Here's how the part is built. I have some questions about the finished solid (model axes, mm). Face numbers are marked on the shaded views. A direction names the side the tool comes from. Coordinates: 2 decimals unless noted, no trailing zeros. Write each loop counter-clockwise with the first axis right and the second up, starting at its lowest first coordinate (ties: lowest second). Pieces come first, ordered by that corner, then holes.
from build123d import *

# Parameters (mm, degrees)
SKETCH1_W             = 44
SKETCH1_H             = 44
BOSS_EXTRUDE1_DEPTH   = 1.2
SKETCH2_W             = 23
SKETCH2_H             = 16
BOSS_EXTRUDE2_DEPTH   = 25
SKETCH3_W             = 7.6
SKETCH3_H             = 10
BOSS_EXTRUDE3_DEPTH   = 10
FILLET1_R             = 1
SKETCH4_W             = 15
SKETCH4_H             = 7.6
BOSS_EXTRUDE4_DEPTH   = 10
CHAMFER2_SIZE         = 3
CHAMFER2_SIZE2        = 0.528980942
CHAMFER2_PART_2_SIZE  = 3
CHAMFER2_PART_2_SIZE2 = 0.528980942
CHAMFER2_PART_3_SIZE  = 3
CHAMFER2_PART_3_SIZE2 = 0.528980942
CHAMFER1_SIZE         = 4
CHAMFER1_SIZE2        = 1.455880937
CHAMFER1_PART_2_SIZE  = 4
CHAMFER1_PART_2_SIZE2 = 1.455880937
CHAMFER1_PART_3_SIZE  = 4
CHAMFER1_PART_3_SIZE2 = 1.455880937
SKETCH5_W             = 15
SKETCH5_H             = 2.1
BOSS_EXTRUDE5_DEPTH   = 8.5
FILLET2_R             = 0.5
SKETCH6_R             = 1.5
CUT_EXTRUDE1_DEPTH    = 2.2


with BuildPart() as part:
    # Sketch1 → Boss-Extrude1 (new body)
    with BuildSketch(Plane(origin=(0, 0, 0), x_dir=(1, 0, 0), z_dir=(0, 1, 0))):
        Rectangle(SKETCH1_W, SKETCH1_H)
    extrude(amount=BOSS_EXTRUDE1_DEPTH)

    # Sketch2 → Boss-Extrude2 (add)
    with BuildSketch(Plane(origin=(0, 1.2, 0), x_dir=(1, 0, 0), z_dir=(0, 1, 0))):
        with Locations((0, 13.5)):
            Rectangle(SKETCH2_W, SKETCH2_H)
    extrude(amount=BOSS_EXTRUDE2_DEPTH)

    # Sketch3 → Boss-Extrude3 (add)
    with BuildSketch(Plane(origin=(0, 1.2, 0), x_dir=(1, 0, 0), z_dir=(0, 1, 0))):
        with Locations((-17.7, -7.5)):
            Rectangle(SKETCH3_W, SKETCH3_H)
    boss_extrude3 = extrude(amount=BOSS_EXTRUDE3_DEPTH)

    # Mirror1: Boss-Extrude3 across plane
    add(boss_extrude3.mirror(Plane(origin=(0, 0, 0), x_dir=(0, 0, 1), z_dir=(1, 0, 0))))

    # Fillet1
    fillet1_edges = [part.edges().sort_by_distance(p)[0] for p in [
        (-11.5, 13.7, -21.5),
        (-11.5, 13.7, -5.5),
        (11.5, 13.7, -5.5),
        (11.5, 13.7, -21.5),
    ]]
    fillet(fillet1_edges, radius=FILLET1_R)

    # Sketch4 → Boss-Extrude4 (add)
    with BuildSketch(Plane(origin=(0, 1.2, 0), x_dir=(1, 0, 0), z_dir=(0, 1, 0))):
        with Locations((-8.2, -17.7)):
            Rectangle(SKETCH4_W, SKETCH4_H)
    extrude(amount=BOSS_EXTRUDE4_DEPTH)

    # Chamfer2
    chamfer2_edges = [part.edges().sort_by_distance(p)[0] for p in [
        (-21.5, 11.2, 7.5),
    ]]
    chamfer2_side = [part.faces().sort_by_distance(p)[0] for p in [
        (-21.5, 6.2, 7.5),
    ]]
    chamfer(chamfer2_edges, length=CHAMFER2_SIZE, length2=CHAMFER2_SIZE2, reference=chamfer2_side[0])

    # Chamfer2 part 2
    chamfer2_part_2_edges = [part.edges().sort_by_distance(p)[0] for p in [
        (21.5, 11.2, 7.5),
    ]]
    chamfer2_part_2_side = [part.faces().sort_by_distance(p)[0] for p in [
        (21.5, 6.2, 7.5),
    ]]
    chamfer(chamfer2_part_2_edges, length=CHAMFER2_PART_2_SIZE, length2=CHAMFER2_PART_2_SIZE2, reference=chamfer2_part_2_side[0])

    # Chamfer2 part 3
    chamfer2_part_3_edges = [part.edges().sort_by_distance(p)[0] for p in [
        (-8.2, 11.2, 21.5),
    ]]
    chamfer2_part_3_side = [part.faces().sort_by_distance(p)[0] for p in [
        (-8.2, 6.2, 21.5),
    ]]
    chamfer(chamfer2_part_3_edges, length=CHAMFER2_PART_3_SIZE, length2=CHAMFER2_PART_3_SIZE2, reference=chamfer2_part_3_side[0])

    # Chamfer1
    chamfer1_edges = [part.edges().sort_by_distance(p)[0] for p in [
        (-13.9, 11.2, 7.5),
    ]]
    chamfer1_side = [part.faces().sort_by_distance(p)[0] for p in [
        (-13.9, 6.2, 7.5),
    ]]
    chamfer(chamfer1_edges, length=CHAMFER1_SIZE, length2=CHAMFER1_SIZE2, reference=chamfer1_side[0])

    # Chamfer1 part 2
    chamfer1_part_2_edges = [part.edges().sort_by_distance(p)[0] for p in [
        (13.9, 11.2, 7.5),
    ]]
    chamfer1_part_2_side = [part.faces().sort_by_distance(p)[0] for p in [
        (13.9, 6.2, 7.5),
    ]]
    chamfer(chamfer1_part_2_edges, length=CHAMFER1_PART_2_SIZE, length2=CHAMFER1_PART_2_SIZE2, reference=chamfer1_part_2_side[0])

    # Chamfer1 part 3
    chamfer1_part_3_edges = [part.edges().sort_by_distance(p)[0] for p in [
        (-8.2, 11.2, 13.9),
    ]]
    chamfer1_part_3_side = [part.faces().sort_by_distance(p)[0] for p in [
        (-8.2, 6.2, 13.9),
    ]]
    chamfer(chamfer1_part_3_edges, length=CHAMFER1_PART_3_SIZE, length2=CHAMFER1_PART_3_SIZE2, reference=chamfer1_part_3_side[0])

    # Sketch5 → Boss-Extrude5 (add)
    with BuildSketch(Plane(origin=(0, 1.2, 0), x_dir=(1, 0, 0), z_dir=(0, 1, 0))):
        with Locations((7.8, -19.95)):
            Rectangle(SKETCH5_W, SKETCH5_H)
    extrude(amount=BOSS_EXTRUDE5_DEPTH)

    # Fillet2
    fillet2_edges = [part.edges().sort_by_distance(p)[0] for p in [
        (0.3, 5.45, 18.9),
        (0.3, 5.45, 21),
        (15.3, 5.45, 21),
        (15.3, 5.45, 18.9),
    ]]
    fillet(fillet2_edges, radius=FILLET2_R)

    # Sketch6 → Cut-Extrude1 (cut, through all)
    with BuildSketch(Plane(origin=(0, 1.2, 0), x_dir=(1, 0, 0), z_dir=(0, 1, 0))):
        with Locations((-18.75, 18.75)):
            Circle(SKETCH6_R)
        with Locations((18.75, 18.75)):
            Circle(SKETCH6_R)
        with Locations((18.75, -18.75)):
            Circle(SKETCH6_R)
        with Locations((-18.75, -18.75)):
            Circle(SKETCH6_R)
    extrude(amount=-CUT_EXTRUDE1_DEPTH, mode=Mode.SUBTRACT)


solid = part.part
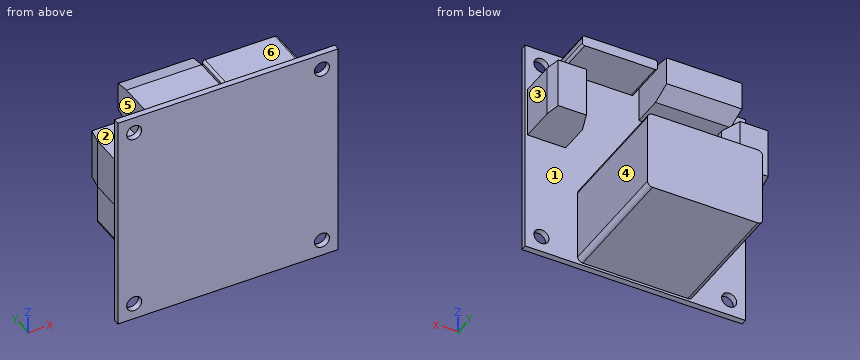
1. I want a section at A-A (z = -18.75). List the corners of the cut face in (x, y) for me, then the cut area to 3 significant figures.
2. If I drill on line 1 (Z direction, x = -18.75, y = 0.5); line 2 (Y direction, x = 12.5, z = -19), over which ranges is the centre line in solid material (lowest first)?
3. I want a section at B-B (x = 18.75). List the corners of the cut face in (y, z) for me.
4. On a 3-axis mill with a long thin cutter (end or side, diameter ignored), from which of +Z, -Z, +X, -X, +Y, -Y can I reach the whole of each face in a straight line? I mean the marked faces 4, 5 and 6. Say none if no direction works.
5. I want a section at C-C (z = -13). List the corners of the cut face in (x, y) for me.
6. Thinking about a two-plate mould opening in X: for the marked faces 1, 2 and 3, which applies, pulls with the +X half, pulls with the -X half, needs draft (parallel to the pull), parting line crosses it, or undercut?
7. For pin 1 Ø10.5 at (x, y) = (0.5, 12) entering from -Z; pin 2 Ø2.5 at (x, y) = (16, 6) entering from -Z; pin 3 Ø5 at (y, z) = (16.5, -9) entering from -X; pin 4 Ø2.5 at (x, z) = (18.75, 18.75) entering from -Y, each with a flat end and sliding along its axis, tell me the tip position at first contact or that it passes through.
8. I want a section at D-D (x = 7). List the corners of the cut face in (y, z) for me, then the cut area to 3 significant figures.
Response values:
1. outline: (-22, 0) - (-20.25, 0) - (-20.25, 1.2) - (-22, 1.2) - close; (-17.25, 0) - (17.25, 0) - (17.25, 1.2) - (11.5, 1.2) - (11.5, 26.2) - (-11.5, 26.2) - (-11.5, 1.2) - (-17.25, 1.2) - close; (20.25, 0) - (22, 0) - (22, 1.2) - (20.25, 1.2) - close
1. area: 621 mm2
2. line 1: z = -22 to -20.25, -17.25 to 17.25, 20.25 to 22
2. line 2: y = 0 to 1.2
3. outline: (0, -22) - (1.2, -22) - (1.2, -20.25) - (0, -20.25) - close; (0, -17.25) - (1.2, -17.25) - (1.2, 2.5) - (11.2, 2.5) - (11.2, 12.5) - (1.2, 12.5) - (1.2, 17.25) - (0, 17.25) - close; (0, 20.25) - (1.2, 20.25) - (1.2, 22) - (0, 22) - close
4. face 4: -Z, +X, +Y
4. face 5: +Z, -X, +Y
4. face 6: +Z, +X, +Y
5. outline: (-22, 0) - (22, 0) - (22, 1.2) - (11.5, 1.2) - (11.5, 26.2) - (-11.5, 26.2) - (-11.5, 1.2) - (-22, 1.2) - close
6. face 1: undercut
6. face 2: needs draft
6. face 3: pulls with the +X half
7. pin 1: stops at z = -21.5
7. pin 2: stops at z = 2.5
7. pin 3: stops at x = -11.5
7. pin 4: passes through
8. outline: (0, -22) - (1.2, -22) - (1.2, -21.5) - (26.2, -21.5) - (26.2, -5.5) - (1.2, -5.5) - (1.2, 18.9) - (9.7, 18.9) - (9.7, 21) - (1.2, 21) - (1.2, 22) - (0, 22) - close
8. area: 471 mm2
